```python
from build123d import *

# Parameters (mm, degrees)
F1_DEPTH = 90


with BuildPart() as f1:
    # F0 (on Front) → F1 (new body)
    with BuildSketch(Plane.XZ):
        Polygon((-2.238045, 9.768403), (-9.738045, 9.768403), (-9.738045, 2.268403), (-7.738045, 2.268403), (-7.738045, 6.35419), (-3.388045, 2.00419), (-3.388045, -0.231597), (-3.388045, -2.467383), (-7.738045, -6.817383), (-7.738045, -2.731597), (-9.738045, -2.731597), (-9.738045, -10.231597), (-2.238045, -10.231597), (-2.238045, -8.231597), (-6.323832, -8.231597), (-1.973832, -3.881597), (2.497741, -3.881597), (6.847741, -8.231597), (2.761955, -8.231597), (2.761955, -10.231597), (10.261955, -10.231597), (10.261955, -2.731597), (8.261955, -2.731597), (8.261955, -6.817383), (3.911955, -2.467383), (3.911955, -0.231597), (3.911955, 2.00419), (8.261955, 6.35419), (8.261955, 2.268403), (10.261955, 2.268403), (10.261955, 9.768403), (2.761955, 9.768403), (2.761955, 7.768403), (6.847741, 7.768403), (2.497741, 3.418403), (-1.973832, 3.418403), (-6.323832, 7.768403), (-2.238045, 7.768403), align=None)
        with BuildLine():
            ThreePointArc((-1.888045, -0.231597), (0.261955, 1.918403), (2.411955, -0.231597))
            ThreePointArc((2.411955, -0.231597), (0.261955, -2.381597), (-1.888045, -0.231597))
        make_face(mode=Mode.SUBTRACT)
    extrude(amount=F1_DEPTH)


solid = f1.part
```
Geometry: final body of the model. Coordinates: model frame, mm. A direction names the side the tool comes from. Coordinates: 2 decimals unless noted, no trailing zeros. Order: outer loops, then holes, each group sorted by start corner. A loop starts at its lowest first (then second) coordinate and runs counter-clockwise, first axis right, second up.
Item 1: Section query A-A (z = -1.5). Output: boundary loops of the cut face in (x, y), then the cut area to 3 significant figures.
Answer:
outline: (-3.39, -90) - (-1.47, -90) - (-1.47, 0) - (-3.39, 0) - close; (2, -90) - (3.91, -90) - (3.91, 0) - (2, 0) - close
area: 345 mm2
Item 2: Access query for faces 4 (the face through (4.642, -44.37, -6.026)), 5 (the face through (2.762, -44, -9)), 6 (the face through (2.762, -44, 9)), 7 (the face through (-3.388, -44, 0)). Directions: +Z, -Z, +X, -X, +Y, -Y. A direction counts if a zero-diameter tool reaches every point of the face in a straight line with its end or side. Return the directions, or none.
Answer:
face 4: +Y, -Y
face 5: -Z, +Y, -Y
face 6: +Z, +Y, -Y
face 7: -X, +Y, -Y
Item 3: Draft query along X for faces 1 (the face through (-9.738, -44, 6)), 2 (the face through (-4.118, -44.37, 5.563)), 3 (the face through (-9, -44, -2.732)). Return one class per face: released by +X, released by -X, zero draft, split by the parting line, or undercut.
Answer:
face 1: released by -X
face 2: undercut
face 3: zero draft
Item 4: Material intervals for line 1 along Z through (x, y) = (3.75, -30); line 2 along X through (y, z) = (-61, 3.75); line 3 along Z through (x, y) = (5, -76.5), sorted ascending.
Answer:
line 1: z = -10.23 to -8.23, -5.13 to 4.67, 7.77 to 9.77
line 2: x = -9.74 to -7.74, -5.13 to -2.31, 2.83 to 5.66, 8.26 to 10.26
line 3: z = -10.23 to -8.23, -6.38 to -3.56, 3.09 to 5.92, 7.77 to 9.77
Item 5: Contact query for flat-ended pins moving along their axis: P1, Ø2, axis at x = 0.5, y = -53.5, coming from the +Z side; P2, Ø3.5, axis at y = -26, z = 0, coming from the +X side. Output: stop coordinate, or through.
Answer:
P1: stops at z = 3.42
P2: stops at x = 3.91
Item 6: Section query B-B (z = 5.5). Output: boundary loops of the cut face in (x, y), then the cut area to 3 significant figures.
Answer:
outline: (-9.74, -90) - (-7.74, -90) - (-7.74, 0) - (-9.74, 0) - close; (-6.88, -90) - (-4.06, -90) - (-4.06, 0) - (-6.88, 0) - close; (4.58, -90) - (7.41, -90) - (7.41, 0) - (4.58, 0) - close; (8.26, -90) - (10.26, -90) - (10.26, 0) - (8.26, 0) - close
area: 869 mm2
